Autodesk Inventor part; units mm, degrees
ref_plane "作業平面4" through (22.5, -5, 0) normal (1, 0, 0) x (0, 0, -1)
ref_plane "作業平面5" through (-23.5, -5, 0) normal (-1, 0, 0) x (0, 0, 1)
ref_plane "作業平面6" through (0, 20, -45) normal (0, 0, 1) x (1, 0, 0)
sketch "スケッチ1" plane through (0, 0, 0) normal (0, 1, 0) x (-1, 0, 0)
  line L0 (11.25, 0) -> (-11.25, 0)
  line L1 (-11.25, 0) -> (-11.25, -120)
  line L2 (-11.25, -120) -> (11.25, -120)
  line L3 (11.25, -120) -> (11.25, 0)
  point P0 (0, 0)
  point P1 (0, 0)
  dimension "d0" = 22.5
  dimension "d3" = 120
extrude "押し出し1" add sketch "スケッチ1" along normal blind 2
sketch "スケッチ2" plane through (0, 0, 0) normal (0, -1, 0) x (1, 0, 0)
  line L0 (19, -120) -> (-19, -120)
  line L1 (-19, -120) -> (-19, -103.05)
  line L2 (-19, -103.05) -> (19, -103.05)
  line L3 (19, -103.05) -> (19, -120)
  line L4 (11.25, -120) -> (-11.25, -120)
  point P0 (0, 0)
  point P1 (0, -120)
  dimension "d6" = 38
  dimension "d11" = 16.95
extrude "押し出し2" add sketch "スケッチ2" against normal blind 13.44
sketch "スケッチ4" plane through (11.25, 0, -103.05) normal (0, 0, 1) x (1, 0, 0)
  circle A0 centre (-11.25, 20) radius 20
  line L0 (7.75, 0) -> (0, 0)
  line L1 (-22.5, 0) -> (0, 0)
  point P0 (-11.25, 0)
  point P1 (-11.25, 0)
  dimension "d12" = 40
extrude "押し出し4" cut sketch "スケッチ4" along normal through all
sketch "スケッチ5" plane through (11.25, 0, -103.05) normal (0, 0, 1) x (1, 0, 0)
  circle A0 centre (-11.25, 20) radius 20
  arc A1 (-11.25, 0) -> (-2.5322, 2) centre (-11.25, 20) ccw
  line L0 (-30.25, 13.44) -> (7.75, 13.44)
  line L1 (7.75, 13.44) -> (7.75, -5)
  line L2 (7.75, -5) -> (-30.25, -5)
  line L3 (-30.25, -5) -> (-30.25, 13.44)
  line L4 (7.75, 0) -> (7.75, 13.44)
  line L5 (7.75, 0) -> (0, 0)
  line L6 (-30.25, 4.22) -> (-11.25, 20)
  line L7 (-11.25, 20) -> (7.75, 4.22)
  point P0 (3.875, 0)
  point P1 (7.6436, 13.44)
  point P2 (-30.1436, 13.44)
  point P3 (7.75, 4.22)
  point P4 (4.1356, 7.2218)
  point P5 (-26.6356, 7.2218)
  point P6 (-3.3514, 13.44)
  point P7 (-19.1486, 13.44)
  dimension "d15" = 5
extrude "押し出し5" add sketch "スケッチ5" along normal up to surface (103.05 mm away) contours A0 L7 L1 L2 L3 L6
sketch "スケッチ24" plane through (11.25, 0, -103.05) normal (0, 0, -1) x (-1, 0, 0)
  line L0 (-7.75, 0) -> (11.25, 0)
  line L1 (-7.75, -5) -> (-7.75, 0)
  line L2 (30.25, -5) -> (-7.75, -5)
  line L3 (30.25, 0) -> (30.25, -5)
  line L4 (11.25, 0) -> (30.25, 0)
  point P0 (11.25, 0)
extrude "押し出し22" add sketch "スケッチ24" along normal up to surface (16.95 mm away)
sketch "スケッチ25" plane through (19, 13.44, -103.05) normal (1, 0, 0) x (0, 0, -1)
  line L0 (-103.05, -13.44) -> (-103.05, -6.2182)
  line L1 (16.95, -18.44) -> (16.95, 0)
  line L2 (16.95, -13.44) -> (-40.05, -13.44)
  line L3 (-40.05, -13.44) -> (-40.05, 1.46)
  line L4 (-40.05, 1.46) -> (16.95, 1.46)
  line L5 (16.95, 1.46) -> (16.95, -13.44)
  dimension "d77" = 14.9
  dimension "d78" = 57
extrude "押し出し23" add sketch "スケッチ25" against normal up to surface (38 mm away)
sketch "スケッチ26" plane through (19, -5, 0) normal (1, 0, 0) x (0, 0, -1)
  line L0 (63, 12.2218) -> (0, 12.2218)
  circle A0 centre (63, 12.2218) radius 12.2218
  line L1 (0, 0) -> (120, 0)
  circle A1 centre (84.1688, 0) radius 12.2218
  line L2 (84.1688, 12.2218) -> (120, 12.2218)
  line L3 (120, 0) -> (120, 19.9)
  point P0 (0, 5)
  point P1 (73.5844, 6.1109)
  point P2 (63, 0)
extrude "押し出し24" cut sketch "スケッチ26" against normal through all contours A1 L1 A0 | A1 L1 | L2 L3 L1 A1 picked at (80.2991, 4.512)
sketch "スケッチ28" plane through (19, -5, 0) normal (1, 0, 0) x (0, 0, -1)
  circle A0 centre (103.05, 29.95) radius 18.95
  line L0 (120, 12.2218) -> (120, 19.9)
  line L1 (120, 19.9) -> (63, 19.9)
  line L2 (84.1688, 12.2218) -> (120, 12.2218)
  point P0 (0, 5)
  point P1 (96.3557, 12.2218)
  point P2 (86.9845, 19.9)
  dimension "d83" = 16.95
  dimension "d84" = 10.05
  dimension "d85" = 37.9
extrude "押し出し25" cut sketch "スケッチ28" against normal through all contours L1 A0 L2 | L1 L0 L2 A0
fillet "フィレット4" radius 2 1 edges at (0, 7.2218, -96.3557)
ref_plane "作業平面4" through (22.5, -5, 0) normal (1, 0, 0) x (0, 0, -1)
ref_plane "作業平面5" through (-23.5, -5, 0) normal (-1, 0, 0) x (0, 0, 1)
sketch "スケッチ29" plane through (22.5, -5, 0) normal (1, 0, 0) x (0, 0, -1)
  line L0 (63, 19.9) -> (63, 9.22)
  line L1 (86.9845, 19.9) -> (63, 19.9)
  arc A0 (84.1688, 12.2218) -> (73.5844, 6.1109) centre (84.1688, 0) ccw
  arc A1 (63, 0) -> (73.5844, 6.1109) centre (63, 12.2218) ccw
  line L2 (63, 9.22) -> (0, 9.22)
  line L3 (63, 9.22) -> (63, -0.3745)
  line L4 (84.1688, 12.2218) -> (84.1688, 19.9)
  point P0 (0, 5)
  point P1 (63, 0)
extrude "押し出し26" add sketch "スケッチ29" against normal up to surface (46 mm away)
fillet "フィレット5" radius 2 4 edges at (19, 11.0609, -84.1688) (19, -0.39, -63) (-19, -0.39, -63) (-19, 11.0609, -84.1688)
ref_plane "作業平面6" through (0, 20, -45) normal (0, 0, 1) x (1, 0, 0)
sketch "スケッチ31" plane through (0, 20, -45) normal (0, 0, 1) x (1, 0, 0)
  circle A0 centre (0, 0) radius 22
  arc A1 (-15.3856, -12.7782) -> (15.3856, -12.7782) centre (0, 0) ccw
  point P0 (0, -20)
  dimension "d95" = 44
extrude "押し出し27" cut sketch "スケッチ31" along normal blind 12
sketch "スケッチ32" plane through (22.5, -5, 0) normal (1, 0, 0) x (0, 0, -1)
  line L0 (63, 19.9) -> (63, 0)
  arc A0 (63, 0) -> (73.5844, 6.1109) centre (63, 12.2218) ccw
  arc A1 (84.1688, 12.2218) -> (73.5844, 6.1109) centre (84.1688, 0) ccw
  line L1 (84.1688, 12.2218) -> (84.1688, 19.9)
  line L2 (84.1688, 19.9) -> (63, 19.9)
  circle A2 centre (103.05, 29.95) radius 4
  circle A3 centre (103.05, 29.95) radius 10
  line L3 (99.5506, 39.3177) -> (106.5494, 20.5823)
  line L4 (106.5494, 20.5823) -> (68.1093, 6.2226)
  line L5 (68.1093, 6.2226) -> (61.1105, 24.9581)
  line L6 (61.1105, 24.9581) -> (99.5506, 39.3177)
  point P0 (0, 5)
  dimension "d98" = 40.05
  dimension "d99" = 10.05
  dimension "d100" = 8
  dimension "d101" = 20
extrude "押し出し28" add sketch "スケッチ32" along normal blind 3.5 contours L5 L4 A1 A0 L0 | L5 L6 A3 L4 L1 L2 | L2 L1 A1 L4 L5 | L3 A2 A3 | A3 L3 A2 | L3 A2 | A2 L3
sketch "スケッチ33" plane through (22.5, -5, 0) normal (-1, 0, 0) x (0, 0, 1)
  line L0 (73.7681, 73.9475) -> (-168.83, 73.9475)
  line L1 (-168.83, 73.9475) -> (-168.83, -57.4645)
  line L2 (-168.83, -57.4645) -> (73.7681, -57.4645)
  line L3 (73.7681, -57.4645) -> (73.7681, 73.9475)
  point P0 (0, 5)
extrude "押し出し29" cut sketch "スケッチ33" along normal through all
sketch "スケッチ34" plane through (22.5, -5, 0) normal (-1, 0, 0) x (0, 0, 1)
  arc A0 (-99.5506, 39.3177) -> (-106.5494, 20.5823) centre (-103.05, 29.95) ccw
  circle A1 centre (-103.05, 29.95) radius 3
  point P0 (0, 5)
  dimension "d106" = 6
extrude "押し出し30" add sketch "スケッチ34" against normal blind 6.5
sketch "スケッチ35" plane through (22.5, -5, 0) normal (-1, 0, 0) x (0, 0, 1)
  circle A0 centre (-67, 6) radius 1.6
  circle A1 centre (-67, 15.9) radius 1.6
  circle A2 centre (-82.1688, 15.9) radius 1.6
  point P0 (0, 5)
extrude "押し出し31" cut sketch "スケッチ35" against normal through all
sketch "スケッチ36" plane through (26, -5, 0) normal (1, 0, 0) x (0, 0, -1)
  line L0 (84.1688, 19.9) -> (63, 19.9)
  line L1 (84.1688, 12.2218) -> (84.1688, 19.9)
  circle A0 centre (82.1688, 15.9) radius 1.35
  circle A1 centre (82.1688, 15.9) radius 4
  line L2 (84.1688, 19.9) -> (88.6672, 13.9022)
  circle A2 centre (67, 6) radius 1.6
  circle A3 centre (67, 15.9) radius 1.6
  circle A4 centre (82.1688, 15.9) radius 1.6
  circle A5 centre (103.05, 29.95) radius 3
  line L3 (99.5506, 39.3177) -> (61.1105, 24.9581)
  line L4 (61.1105, 24.9581) -> (63, 19.9)
  line L5 (63, 19.9) -> (63, 0)
  arc A6 (63, 0) -> (73.5844, 6.1109) centre (63, 12.2218) ccw
  arc A7 (84.1688, 12.2218) -> (73.5844, 6.1109) centre (84.1688, 0) ccw
  line L6 (84.1688, 12.2218) -> (106.5494, 20.5823)
  arc A8 (106.5494, 20.5823) -> (99.5506, 39.3177) centre (103.05, 29.95) ccw
  circle A9 centre (103.05, 29.95) radius 5
  circle A10 centre (103.05, 29.95) radius 3
  point P0 (0, 5)
  point P1 (82.1688, 19.9)
  point P2 (85.3688, 18.3)
  dimension "d111" = 10
extrude "押し出し32" cut sketch "スケッチ36" against normal blind 2 contours L1 A1 L0 | L2 A1 L1 | L0 L4 L3 A8 L6 L2
fillet "フィレット6" radius 2 3 edges at (24, 14.4777, -83.9577) (24, 11.1011, -87.018) (24, 14.9, -72.5844)
fillet "フィレット7" radius 10 1 edges at (23.25, 19.9581, -61.1105)
properties part number "fore_arm_side_left"
Could you check a few things on this model? Use its own coordinates, in mm. A direction names the side the tool comes from. Coordinates: 2 decimals unless noted, no trailing zeros. Loops run counter-clockwise (first coordinate to the right, second up) from the corner with the lowest first, then second, coordinate; pieces in that order, holes last. Notation, with made-up numbers: (58, 47) -> (93, 47) arc R16 ccw to (93, 60) -> close; hole circle Ø8 at (73.5, 77). An arc over 180 degrees is marked (long way). Answer in a Markdown table with one row per item.
(1) If I drill on probe 1 along X at (y, z) = (21.5, -108); probe 2 along Y at (x, z) = (25, -83.5); probe 3 along Y at (x, z) = (25.25, -67), over which ranges is the centre line in solid material (lowest first)?
Results found:
| item | result |
|---|---|
| probe 1 | x = 22.5 to 24 |
| probe 2 | y = 7.2 to 10.01, 11.79 to 14.95 |
| probe 3 | y = -4.33 to -0.6, 2.6 to 9.3, 12.5 to 15.05 |
(2) Imagine slicing it at C-C (z = -105.5). List the corners of the cut face in (x, y) for me.
Results found:
| item | result |
|---|---|
| outline | (22.5, 15.19) -> (24, 15.19) -> (24, 20.59) -> (26, 20.59) -> (26, 23.22) -> (29, 23.22) -> (29, 26.68) -> (26, 26.68) -> (26, 29.31) -> (24, 29.31) -> (24, 34.65) -> (22.5, 34.65) -> close |
(3) Thinking about a two-plate mould opening in Y: for faces 1 (the face through (24.6, 15.47, -72.72)), 2 (the face through (23.24, 28.65, -112.34)), 3 (the face through (24.226, 10.97, -83.767)), which applies, released by +Y, released by -Y, zero draft, split by the parting line, or undercut?
Results found:
| item | result |
|---|---|
| face 1 | released by +Y |
| face 2 | split by the parting line |
| face 3 | undercut |
(4) Will these pins go through, and if not, where does the flat tip stop? pin 1 Ø6 at (y, z) = (7, -75.5) entering from +X; pin 2 Ø1 at (x, y) = (25, 17.5) entering from +Z; pin 3 Ø1.5 at (x, z) = (24, -108) entering from -Y.
Results found:
| item | result |
|---|---|
| pin 1 | stops at x = 26 |
| pin 2 | passes through |
| pin 3 | stops at y = 15.87 |
(5) Imagine slicing it at A-A (x = 24.75). List the corners of the cut face in (y, z) for me.
Results found:
| item | result |
|---|---|
| outline | (-5, -63) arc R12.22 ccw to (1.11, -73.58) arc R12.22 cw to (7.22, -84.17) -> (9.06, -89.1) -> (13.56, -85.72) arc R4.44 ccw to (15.34, -82.17) -> (15.34, -63.06) arc R10 ccw to (14.9, -63) -> close; circle Ø10 at (24.95, -103.05); hole circle Ø3.2 at (1, -67); hole circle Ø3.2 at (10.9, -82.17); hole circle Ø3.2 at (10.9, -67) |
(6) Imagine slicing it at B-B (y = 2). List the corners of the cut face in (x, z) for me.
Results found:
| item | result |
|---|---|
| outline | (22.5, -74.15) -> (26, -74.15) -> (26, -68.25) -> (22.5, -68.25) -> close; (22.5, -65.75) -> (26, -65.75) -> (26, -63) -> (22.5, -63) -> close |
(7) Imagine slicing it at D-D (y = 24.95). List the corners of the cut face in (x, z) for me, plus the area to 3 significant figures.
Results found:
| item | result |
|---|---|
| outline | (22.5, -113.05) -> (24, -113.05) -> (24, -108.05) -> (26, -108.05) -> (26, -106.05) -> (29, -106.05) -> (29, -100.05) -> (26, -100.05) -> (26, -98.05) -> (24, -98.05) -> (24, -74.47) -> (22.5, -74.47) -> close |
| area | 95.9 mm^2 |
(8) For faces 4 (the face through (24, 22, -93)), 5 (the face through (23.45, 10.53, -93.03)), which set-ups out of +Z, -Z, +X, -X, +Y, -Y let a thin tool reach every point of the face, with its end or its side?
Results found:
| item | result |
|---|---|
| face 4 | +X |
| face 5 | -Z, +X, -X, -Y |
